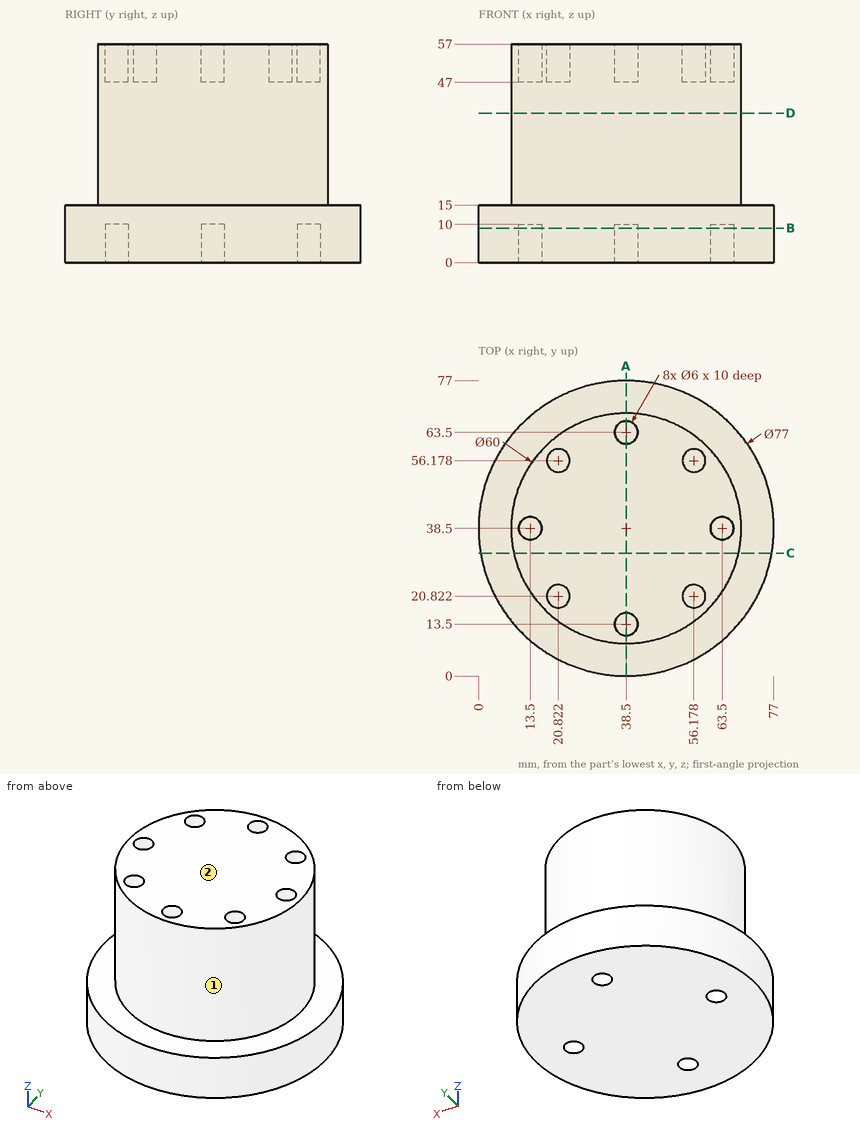
Job drawing, mm, ordinate dimensions from the low corner. One solid piece. A direction names the side the tool comes from. Coordinates: 2 decimals unless noted, no trailing zeros. Order: outer loops, then holes, each group sorted by start corner. A loop starts at its lowest first (then second) coordinate and runs counter-clockwise, first axis right, second up. Notation, with made-up numbers: (57.5, -22.5) -> (109.5, -22.5) arc R4 ccw to (109.5, -16.5) -> close; hole circle Ø4 at (-38.75, 32). An arc over 180 degrees is marked (long way). Return JSON: item names as keys, results as strings. Group by question number.
Item 1: Flat gauge pins, fed straight in: P1, Ø8, axis at y = 9.5, z = 45, coming from the +X side; P2, Ø3, axis at x = 67, y = 64, coming from the +Z side; P3, Ø1.8, axis at x = 56.5, y = 57.5, coming from the +Z side. Where does each tip first touch, or does it go through?
Item 2: Saw through at A-A on x = 38.5. Write the cut outline in (y, z).
Item 3: Tool access for the marked faces 1 and 2: list every direction of +Z, -Z, +X, -X, +Y, -Y with a clear straight run to the whole face (end or side of a thin tool).
Item 4: Wall check: line 1 along Y through (x, z) = (38.5, 4.5); line 2 along Y through (x, z) = (38.5, 51.5); line 3 along Z through (x, y) = (19, 12). Give the ranges that are in metal, low to high. Write a range as [from, to].
Item 5: Saw through at B-B on z = 9. Write the cut outline in (x, y).
Item 6: Saw through at C-C on y = 32. Write the cut outline in (x, z).
Item 7: Saw through at D-D on z = 39. Write the cut outline in (x, y).
Values found:
{
 "1": {"P1": "stops at x = 55.08", "P2": "stops at z = 15", "P3": "stops at z = 47"},
 "2": {"outline": "(0, 0) -> (10.5, 0) -> (10.5, 10) -> (16.5, 10) -> (16.5, 0) -> (60.5, 0) -> (60.5, 10) -> (66.5, 10) -> (66.5, 0) -> (77, 0) -> (77, 15) -> (68.5, 15) -> (68.5, 57) -> (66.5, 57) -> (66.5, 47) -> (60.5, 47) -> (60.5, 57) -> (16.5, 57) -> (16.5, 47) -> (10.5, 47) -> (10.5, 57) -> (8.5, 57) -> (8.5, 15) -> (0, 15) -> close"},
 "3": {"face 1": "+Z", "face 2": "+Z, +X, -X, +Y, -Y"},
 "4": {"line 1": "y = [0, 10.5], [16.5, 60.5], [66.5, 77]", "line 2": "y = [8.5, 10.5], [16.5, 60.5], [66.5, 68.5]", "line 3": "z = [0, 15]"},
 "5": {"outline": "circle Ø77 at (38.5, 38.5); hole circle Ø6 at (13.5, 38.5); hole circle Ø6 at (38.5, 13.5); hole circle Ø6 at (38.5, 63.5); hole circle Ø6 at (63.5, 38.5)"},
 "6": {"outline": "(0.55, 0) -> (76.45, 0) -> (76.45, 15) -> (67.79, 15) -> (67.79, 57) -> (9.21, 57) -> (9.21, 15) -> (0.55, 15) -> close"},
 "7": {"outline": "circle Ø60 at (38.5, 38.5)"}
}
